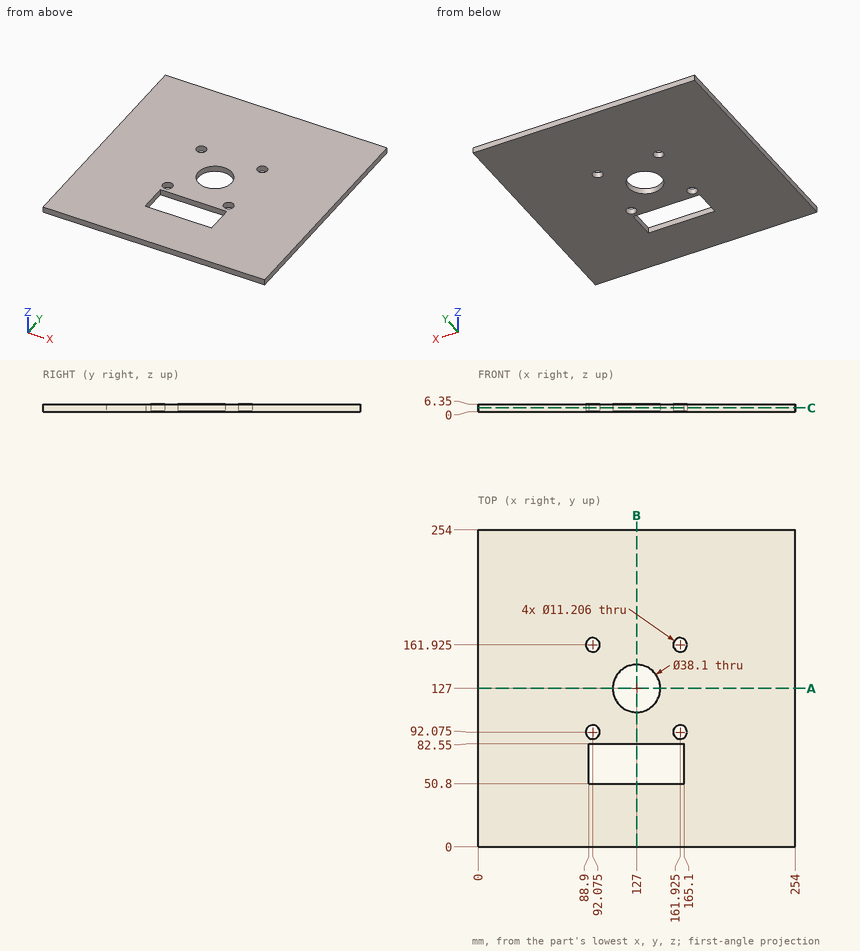
Input: dimensioned drawing with shaded views. Units: mm. Origin: part minimum x, y, z. Give positions to 0.01 mm unless a question says otherwise; leave off trailing zeros. Write each loop counter-clockwise with the first axis right and the second up, starting at its lowest first coordinate (ties: lowest second). Pieces come first, ordered by that corner, then holes.
1. Section query B-B, the plane x = 127. Return loops of the section in (y, z), then the cut area to 3 significant figures.
2. Section query C-C, the plane z = 3.25. Count the separate pieces of the cut face and the enclosed holes in it, then the cut area to 3 significant figures.
3. Pin query (flat end, axial travel): P1, Ø6.5, axis at x = 161.925, y = 161.925, coming from the +Z side. Return the tip coordinate at first contact, or that it passes through.
4. Section query A-A, the plane y = 127. Return loops of the section in (x, z), then the cut area to 3 significant figures.
5. Line query: probe 1 along Y at (x, z) = (127, 2.25); probe 2 along X at (y, z) = (62, 5.25); probe 3 along X at (y, z) = (90.5, 5.25). Output: solid intervals per line, ascending.
Computed:
1. outline: (0, 0) - (50.8, 0) - (50.8, 6.35) - (0, 6.35) - close; (82.55, 0) - (107.95, 0) - (107.95, 6.35) - (82.55, 6.35) - close; (146.05, 0) - (254, 0) - (254, 6.35) - (146.05, 6.35) - close
1. area: 1,170 mm2
2. separate pieces: 1
2. enclosed holes: 6
2. area: 60,600 mm2
3. P1: passes through
4. outline: (0, 0) - (107.95, 0) - (107.95, 6.35) - (0, 6.35) - close; (146.05, 0) - (254, 0) - (254, 6.35) - (146.05, 6.35) - close
4. area: 1,370 mm2
5. probe 1: y = 0 to 50.8, 82.55 to 107.95, 146.05 to 254
5. probe 2: x = 0 to 88.9, 165.1 to 254
5. probe 3: x = 0 to 86.7, 97.45 to 156.55, 167.3 to 254
